from build123d import *

# Parameters (mm, degrees)
SKETCH1_W           = 40
SKETCH1_H           = 3
SKETCH1_W_2         = 10
SKETCH1_H_2         = 7
BOSS_EXTRUDE1_DEPTH = 26
SKETCH3_R           = 1.725
SKETCH3_W           = 4
SKETCH3_H           = 8
CUT_EXTRUDE1_DEPTH  = 49.744230428
SKETCH4_R           = 3
CUT_EXTRUDE2_DEPTH  = 4


with BuildPart() as part:
    # Sketch1 → Boss-Extrude1 (new body)
    with BuildSketch(Plane.XY):
        with Locations((20, 1.5)):
            Rectangle(SKETCH1_W, SKETCH1_H)
        Polygon((40, 3), (10, 10), (10, 3), align=None)
        with Locations((5, 6.5)):
            Rectangle(SKETCH1_W_2, SKETCH1_H_2)
    extrude(amount=BOSS_EXTRUDE1_DEPTH)

    # Sketch3 → Cut-Extrude1 (cut, through all)
    with BuildSketch(Plane.XZ):
        with Locations(Location((7.5, 21.8, 0), (0, 0, 270))):
            Circle(SKETCH3_R)
        with Locations(Location((7.5, 4.2, 0), (0, 0, 270))):
            Circle(SKETCH3_R)
        with Locations((7.75, 13)):
            Rectangle(SKETCH3_W, SKETCH3_H)
    extrude(amount=-CUT_EXTRUDE1_DEPTH, mode=Mode.SUBTRACT)

    # Sketch4 → Cut-Extrude2 (cut)
    with BuildSketch(Plane(origin=(0, 10, 0), x_dir=(1, 0, 0), z_dir=(0, 1, 0))):
        with Locations(Location((7.5, -4.2, 0), (0, 0, 180))):
            Circle(SKETCH4_R)
        with Locations(Location((7.5, -21.8, 0), (0, 0, 180))):
            Circle(SKETCH4_R)
    extrude(amount=-CUT_EXTRUDE2_DEPTH, mode=Mode.SUBTRACT)


solid = part.part
The listing builds one solid part. Answer for the finished solid, in the listing's coordinates (mm). A direction names the side the tool comes from. Round coordinates to 2 decimals unless told otherwise and drop trailing zeros. Loops run counter-clockwise (first coordinate to the right, second up) from the corner with the lowest first, then second, coordinate; pieces in that order, holes last. Notation, with made-up numbers: M -30,42.5 L 4,42.5 A17 cw 4,56.5 Z; hole C 59.25,-6.5 d9. An arc over 180 degrees is marked long. Return JSON: item names as keys, results as strings.
Q1. Find section D-D, the plane z = 21.8. Determine the outline of the cut face in (x, y) (3 decimals), plus the area to 3 significant figures.
Results list:
{"outline": "M 0,0 L 5.775,0 L 5.775,6 L 4.5,6 L 4.5,10 L 0,10 Z; M 9.225,0 L 40,0 L 40,3 L 10.5,9.883 L 10.5,6 L 9.225,6 Z", "area": "250 mm2"}
Q2. Find section C-C, the plane y = 8.25. Determine the outline of the cut face in (x, z), plus the area to 3 significant figures.
Results list:
{"outline": "M 0,0 L 17.5,0 L 17.5,26 L 0,26 Z; hole C 7.5,4.2 d6; hole C 7.5,21.8 d6; hole M 5.75,9 L 9.75,9 L 9.75,17 L 5.75,17 Z", "area": "366 mm2"}
Q3. Which of the six approach directions +Z, -Z, +X, -X, +Y, -Y give full straight-line access (tool end or side, diameter ignored) to faces 4 (the face through (8, 5, 17)), 5 (the face through (7.5, 6, 19.8)), 6 (the face through (20, 0, 13))?
Results list:
{"face 4": "+Y, -Y", "face 5": "+Y", "face 6": "+Z, -Z, +X, -X, -Y"}
Q4. Find section B-B, the plane z = 11.75. Determine the outline of the cut face in (x, y).
Results list:
{"outline": "M 0,0 L 5.75,0 L 5.75,10 L 0,10 Z; M 9.75,0 L 40,0 L 40,3 L 10,10 L 9.75,10 Z"}
Q5. Each of these flat-tipped pins is pushed along its axis until it touches: pin 1 Ø1.5 at (x, z) = (18, 15) entering from +Y; pin 2 Ø3 at (x, z) = (7.5, 21.8) entering from +Y; pin 3 Ø5.5 at (x, z) = (7.5, 4.2) entering from +Y; pin 4 Ø10 at (x, z) = (21, 14) entering from +Y. Where does it stop, or does it pass through?
Results list:
{"pin 1": "stops at y = 8.31", "pin 2": "passes through", "pin 3": "stops at y = 6", "pin 4": "stops at y = 8.6"}
Q6. The mould has two halves that part along Z. Classify faces 1 (the face through (9.21, 2.96, 4.42)), 2 (the face through (15, 4, 0)), 3 (the face through (0, 5, 13)): released by +Z, released by -Z, zero draft, split by the parting line, or undercut.
Results list:
{"face 1": "undercut", "face 2": "released by -Z", "face 3": "zero draft"}
Q7. Find the intervals of material crossed by line 1 along Z through (x, y) = (7.5, 8.35); line 2 along X through (y, z) = (2.65, 4.2) (3 decimals); line 3 along X through (y, z) = (2.5, 3), in increasing order. Write a range as from..to.
Results list:
{"line 1": "z = 0..1.2, 7.2..9, 17..18.8, 24.8..26", "line 2": "x = 0..5.775, 9.225..40", "line 3": "x = 0..6.26, 8.74..40"}
Q8. Find section A-A, the plane x = 7.5. Determine the outline of the cut face in (y, z) (3 decimals).
Results list:
{"outline": "M 0,0 L 10,0 L 10,1.2 L 6,1.2 L 6,2.475 L 0,2.475 Z; M 0,5.925 L 6,5.925 L 6,7.2 L 10,7.2 L 10,9 L 0,9 Z; M 0,17 L 10,17 L 10,18.8 L 6,18.8 L 6,20.075 L 0,20.075 Z; M 0,23.525 L 6,23.525 L 6,24.8 L 10,24.8 L 10,26 L 0,26 Z"}
